from build123d import *
from build123d.topology import SkipClean

# Parameters (mm, degrees)
BOSS_EXTRU_1_DEPTH            = 3.9
BOSS_EXTRU_2_START            = 2
ESQUISSE2_R                   = 7.3
BOSS_EXTRU_2_DEPTH            = 2
D_GAGEMENT_M31_D              = 3.2
DIAM_TRE_DU_PER_AGE_3_0_3_1_D = 3
ESQUISSE6_R                   = 2.75
ENL_V_MAT_EXTRU_1_DEPTH       = 3.4
ESQUISSE9_R                   = 3.75
ENL_V_MAT_EXTRU_2_DEPTH       = 1.2
ENL_V_MAT_EXTRU_3_DEPTH       = 30.057701217
ENL_V_MAT_EXTRU_4_DEPTH       = 4.8
ENL_V_MAT_EXTRU_5_DEPTH       = 29.718460962
ENL_V_MAT_EXTRU_5_DEPTH_BACK  = 29.718460962
ESQUISSE14_R                  = 1


with BuildPart() as part:
    # Esquisse1 → Boss.-Extru.1 (new body)
    with BuildSketch(Plane(origin=(0, 0, 0), x_dir=(1, 0, 0), z_dir=(0, 1, 0))):
        with BuildLine():
            Line((-10.433120339, 3.8), (-23.7, 3.8))
            ThreePointArc((-23.7, 3.8), (-27.5, 0), (-23.7, -3.8))
            Line((-23.7, -3.8), (-10.433120339, -3.8))
            ThreePointArc((-10.433120339, -3.8), (-7.252616143, -4.319261998), (-4.402414941, -5.823121387))
            ThreePointArc((-4.402414941, -5.823121387), (7.3, 0), (-4.402414941, 5.823121387))
            ThreePointArc((-4.402414941, 5.823121387), (-7.252616143, 4.319261998), (-10.433120339, 3.8))
        make_face()
    extrude(amount=BOSS_EXTRU_1_DEPTH)

    # Esquisse2 → Boss.-Extru.2 (add)
    with SkipClean():  # the faces are left unmerged after this step: merging them gives an invalid solid
        with BuildSketch(Plane(origin=(0, 0, 0), x_dir=(-1, 0, 0), z_dir=(0, -1, 0)).offset(BOSS_EXTRU_2_START)):
            with Locations(Location((0, 0, 0), (0, 0, 90))):
                Circle(ESQUISSE2_R)
            with BuildLine():
                Line((23.7, -2.8), (19.8, -2.8))
                ThreePointArc((19.8, -2.8), (17, 0), (19.8, 2.8))
                Line((19.8, 2.8), (23.7, 2.8))
                ThreePointArc((23.7, 2.8), (26.5, 0), (23.7, -2.8))
            make_face()
        extrude(amount=-BOSS_EXTRU_2_DEPTH)

    # D_gagement M31 (through all)
    with Locations(Plane(origin=(0, 3.9, 0), x_dir=(1, 0, 0), z_dir=(0, 1, 0))):
        with Locations((0, 0)):
            Hole(D_GAGEMENT_M31_D / 2)

    # Diam_tre du per_age _3.0 _3_1 (through all)
    with Locations(Plane(origin=(0, -2, 0), x_dir=(-1, 0, 0), z_dir=(0, -1, 0))):
        with Locations((19.75, 0), (23.75, 0)):
            Hole(DIAM_TRE_DU_PER_AGE_3_0_3_1_D / 2)

    # Esquisse6 → Enl_v. mat.-Extru.1 (cut)
    with SkipClean():  # the faces are left unmerged after this step: merging them gives an invalid solid
        with BuildSketch(Plane.XZ.offset(2)):
            with Locations(Location((0, 0, 0), (0, 0, 270))):
                Circle(ESQUISSE6_R)
        extrude(amount=-ENL_V_MAT_EXTRU_1_DEPTH, mode=Mode.SUBTRACT)

    # Esquisse9 → Enl_v. mat.-Extru.2 (cut)
    with SkipClean():  # the faces are left unmerged after this step: merging them gives an invalid solid
        with BuildSketch(Plane(origin=(0, 3.9, 0), x_dir=(1, 0, 0), z_dir=(0, 1, 0))):
            with Locations(Location((0, 0, 0), (0, 0, 270))):
                Circle(ESQUISSE9_R)
        extrude(amount=-ENL_V_MAT_EXTRU_2_DEPTH, mode=Mode.SUBTRACT)

    # Esquisse10 → Enl_v. mat.-Extru.3 (cut, through all)
    with SkipClean():  # the faces are left unmerged after this step: merging them gives an invalid solid
        with BuildSketch(Plane(origin=(0, 3.9, 0), x_dir=(1, 0, 0), z_dir=(0, 1, 0))):
            with BuildLine():
                Line((-8.533974596, 0.5), (7.987060463, 0.5))
                Line((7.987060463, 0.5), (7.987060463, -0.5))
                Line((7.987060463, -0.5), (-8.533974596, -0.5))
                ThreePointArc((-8.533974596, -0.5), (-10.4, 0), (-8.533974596, 0.5))
            make_face()
        extrude(amount=-ENL_V_MAT_EXTRU_3_DEPTH, mode=Mode.SUBTRACT)

    # Esquisse11 → Enl_v. mat.-Extru.4 (cut)
    with SkipClean():  # the faces are left unmerged after this step: merging them gives an invalid solid
        with BuildSketch(Plane.XZ.offset(2)):
            with BuildLine():
                Line((2.5, 6.85857128), (2.5, 4.5))
                ThreePointArc((2.5, 4.5), (3.085786438, 3.085786438), (4.5, 2.5))
                Line((4.5, 2.5), (6.85857128, 2.5))
                ThreePointArc((6.85857128, 2.5), (5.161879503, 5.161879503), (2.5, 6.85857128))
            make_face()
            with BuildLine():
                Line((-2.5, -4.5), (-2.5, -6.85857128))
                Line((-2.5, -6.85857128), (-4.5, -6.85857128))
                Line((-4.5, -6.85857128), (-9.098379022, -3.889477026))
                ThreePointArc((-9.098379022, -3.889477026), (-8.17646592, -2.875581558), (-6.85857128, -2.5))
                Line((-6.85857128, -2.5), (-4.5, -2.5))
                ThreePointArc((-4.5, -2.5), (-3.085786438, -3.085786438), (-2.5, -4.5))
            make_face()
        extrude(amount=-ENL_V_MAT_EXTRU_4_DEPTH, mode=Mode.SUBTRACT)

    # Esquisse14 → Enl_v. mat.-Extru.5 (cut, two sides: drawn at the far end of the back side and taken through both)
    with SkipClean():  # the faces are left unmerged after this step: merging them gives an invalid solid
        with BuildSketch(Plane.XY.offset(-ENL_V_MAT_EXTRU_5_DEPTH_BACK)):
            with Locations((5, 0.4)):
                Circle(ESQUISSE14_R)
            with Locations(Location((-5, 0.4, 0), (0, 0, 60))):
                Circle(ESQUISSE14_R)
        extrude(amount=ENL_V_MAT_EXTRU_5_DEPTH + ENL_V_MAT_EXTRU_5_DEPTH_BACK, mode=Mode.SUBTRACT)


solid = part.part
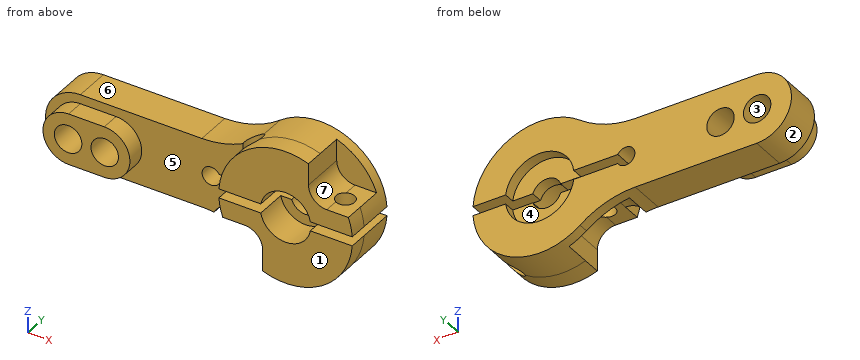
Verification items for the finished model (mm, model axes). Face numbers are marked on the shaded views. A direction names the side the tool comes from. Coordinates: 2 decimals unless noted, no trailing zeros. Order: outer loops, then holes, each group sorted by start corner. A loop starts at its lowest first (then second) coordinate and runs counter-clockwise, first axis right, second up. Notation, with made-up numbers: (35.5, 55.25) -> (88.5, 55.25) arc R17 cw to (88.5, 62.25) -> close; hole circle Ø11 at (-15, 42). An arc over 180 degrees is marked (long way). Put each result on its own line as item: value. Start each with the question number.
1. Go/stop test with flat-tipped pins: pin 1 Ø2.5 at (x, z) = (-23.75, 0) entering from +Y; pin 2 Ø1.2 at (y, z) = (1, 6) entering from +X; pin 3 Ø1.8 at (x, z) = (1, -1) entering from -Y; pin 4 Ø3 at (x, y) = (-4, 1) entering from +Z. Record where each tip stops, or that it passes through.
2. Material ranges on L1, parallel to X at y = 2.3, z = -0.25; L2, parallel to Y at x = -5, z = -2.25; L3, parallel to X at y = 0.4, z = -2.25, recorded low to high. Write a range as [from, to].
3. Cross-section at A-A, the plane z = 0. Record the boundary of the cut face in (x, y).
4. Access from +Z, -Z, +X, -X, +Y, -Y to the whole of each face (thin tool, end or side, straight path). Record for the marked faces 5, 6 and 7.
5. Cross-section at B-B, the plane y = -1.6. Record the boundary of the cut face in (x, z), then the cut area to 3 significant figures.
6. Cross-section at C-C, the plane x = -9.5. Record the boundary of the cut face in (y, z).
7. Mould release check, pull along X, two halves, no side actions. Record for the marked faces 1, 2, 3 and 4: released by +X, released by -X, zero draft, split by the parting line, or undercut.
8. Cross-section at D-D, the plane y = 3.4. Record the boundary of the cut face in (x, z), then the cut area to 3 significant figures.
Computed:
1. pin 1: through
1. pin 2: x = 2.5
1. pin 3: y = 1.4
1. pin 4: z = 6.86
2. L1: [-27.49, -25.23], [-22.27, -21.23], [-18.27, -10.37]
2. L2: [-2, -0.6], [1.4, 3.9]
2. L3: [-26.76, -6], [-4, -1.58], [1.58, 4], [6, 6.94]
3. outline: (-27.5, 0) -> (-26.5, 0) -> (-26.5, -2) -> (-25.25, -2) -> (-25.25, 3.9) -> (-27.5, 3.9) -> close; (-22.25, -2) -> (-21.25, -2) -> (-21.25, 3.9) -> (-22.25, 3.9) -> close; (-18.25, -2) -> (-17, -2) -> (-17, 0) -> (-10.4, 0) -> (-10.4, 3.9) -> (-18.25, 3.9) -> close
4. face 5: -Y
4. face 6: +Z, -X, +Y, -Y
4. face 7: +Z, +X, -Y
5. outline: (-23.7, -2.8) -> (-19.8, -2.8) arc R2.8 ccw to (-19.8, 2.8) -> (-23.7, 2.8) arc R2.8 ccw to start; (-7.28, -0.5) arc R7.3 ccw to (-6.86, -2.5) -> (-4.5, -2.5) arc R2 cw to (-2.5, -4.5) -> (-2.5, -6.86) arc R7.3 ccw to (7.28, -0.5) -> (2.7, -0.5) arc R2.75 cw to (-2.7, -0.5) -> close; (-7.28, 0.5) -> (-2.7, 0.5) arc R2.75 cw to (2.7, 0.5) -> (7.28, 0.5) arc R7.3 ccw to (6.86, 2.5) -> (4.5, 2.5) arc R2 cw to (2.5, 4.5) -> (2.5, 6.86) arc R7.3 ccw to start; hole circle Ø3 at (-23.75, 0); hole circle Ø3 at (-19.75, 0)
5. area: 144 mm2
6. outline: (0, -3.84) -> (3.9, -3.84) -> (3.9, -0.99) -> (0, -0.99) -> close; (0, 0.99) -> (3.9, 0.99) -> (3.9, 3.84) -> (0, 3.84) -> close
7. face 1: zero draft
7. face 2: released by -X
7. face 3: undercut
7. face 4: undercut
8. outline: (-23.7, -3.8) -> (-10.43, -3.8) arc R10 cw to (-4.4, -5.82) arc R7.3 ccw to (7.28, -0.5) -> (3.72, -0.5) arc R3.75 cw to (-3.72, -0.5) -> (-8.53, -0.5) arc R1 cw (long way) to (-8.53, 0.5) -> (-3.72, 0.5) arc R3.75 cw to (3.72, 0.5) -> (7.28, 0.5) arc R7.3 ccw to (-4.4, 5.82) arc R10 cw to (-10.43, 3.8) -> (-23.7, 3.8) arc R3.8 ccw to start; hole circle Ø3 at (-23.75, 0); hole circle Ø3 at (-19.75, 0)
8. area: 251 mm2
